from build123d import *

# Parameters (mm, degrees)
F0_R     = 38.1
F1_DEPTH = 76.2
F2_R     = 31.75
F3_DEPTH = 19.05
F4_R     = 5.08
F6_D     = 7.62
F6_DEPTH = 21.59
F6_TIP   = 2.2892789585
F7_D     = 60.96
F7_DEPTH = 55.88
F7_TIP   = 18.314231668


with BuildPart() as f1:
    # F0 (on Front) → F1 (new body)
    with BuildSketch(Plane.XZ):
        Circle(F0_R)
    extrude(amount=F1_DEPTH)

    # F2 (on Front) → F3 (join)
    with BuildSketch(Plane.XZ):
        Circle(F2_R)
    extrude(amount=-F3_DEPTH)

    # F4
    f4_edges = [f1.edges().sort_by_distance(p)[0] for p in [
        (-31.75, 19.05, 0),
        (38.1, -38.1, 0),
        (-38.1, 0, 0),
        (-38.1, -76.2, 0),
    ]]
    fillet(f4_edges, radius=F4_R)

    # F6 (one way)
    with BuildSketch(Plane.XZ):
        with Locations((0, 0)):
            Circle(F6_D / 2)
    extrude(amount=-F6_DEPTH, mode=Mode.SUBTRACT)
    with Locations(Plane.XZ):
        with Locations((0, 0)):
            with Locations((0, 0, -(F6_DEPTH + F6_TIP / 2))):  # 118° drill point
                Cone(0, F6_D / 2, F6_TIP, mode=Mode.SUBTRACT)

    # F7 (one way)
    with BuildSketch(Plane(origin=(0, 0, 0), x_dir=(1, 0, 0), z_dir=(0, 1, 0))):
        with Locations((0, 0)):
            Circle(F7_D / 2)
    extrude(amount=-F7_DEPTH, mode=Mode.SUBTRACT)
    with Locations(Plane(origin=(0, 0, 0), x_dir=(1, 0, 0), z_dir=(0, 1, 0))):
        with Locations((0, 0)):
            with Locations((0, 0, -(F7_DEPTH + F7_TIP / 2))):  # 118° drill point
                Cone(0, F7_D / 2, F7_TIP, mode=Mode.SUBTRACT)


solid = f1.part
Read the model definition and answer for the solid it produces. Units are mm, in the model's axes. A direction names the side the tool comes from. Round coordinates to 2 decimals unless told otherwise and drop trailing zeros. Loops run counter-clockwise (first coordinate to the right, second up) from the corner with the lowest first, then second, coordinate; pieces in that order, holes last.
Q1. Section A-A on y = 6 is taken. Write down the section's boundary in (x, z).
Q2. Consider probe 1 along Z at (x, y) = (0, -40); probe 2 along Z at (x, y) = (0, 14); probe 3 along X at (y, z) = (-23.5, -1). Determine where each line is inside the solid, lowest interval first.
Q3. Determine the mould class of faces 1 (the face through (-30.235, -37.638, -23.183)), 2 (the face through (5.049, -71.014, -1.59)), 3 (the face through (-17, 0, 27)) for opening direction Z: released by +Z, released by -Z, zero draft, split by the parting line, or undercut.
Q4. Each of these flat-tipped pins is pushed along its axis until it touches: pin 1 (4 mm diameter, centred on y = -26, z = -25.5, fed in from -X); pin 2 (10 mm diameter, centred on x = 5, y = -8, fed in from -Z); pin 3 (5 mm diameter, centred on x = -28.5, z = -23.5, fed in from -Y); pin 4 (10 mm diameter, centred on x = 0, z = 0, fed in from +Y). Where does it stop, or does it pass through?
Q5. Which of the six approach directions +Z, -Z, +X, -X, +Y, -Y give full straight-line access (tool end or side, diameter ignored) to faces 4 (the face through (6, 0, 0)), 5 (the face through (-0.83, 9.39, -3.72)), 6 (the face through (0, -76.2, 0))?
Q6. Section B-B on y = -21.5 is taken. Write down the section's boundary in (x, z), and give its area (3 significant figures).
Output:
1. outline: circle Ø63.5 at (0, 0); hole circle Ø7.62 at (0, 0)
2. probe 1: z = -38.1 to -30.48, 30.48 to 38.1
2. probe 2: z = -31.75 to -3.81, 3.81 to 31.75
2. probe 3: x = -38.09 to -30.46, 30.46 to 38.09
3. face 1: split by the parting line
3. face 2: undercut
3. face 3: zero draft
4. pin 1: stops at x = -29.99
4. pin 2: stops at z = -38.1
4. pin 3: stops at y = -76
4. pin 4: stops at y = 19.05
5. face 4: none
5. face 5: +Y
5. face 6: +Z, -Z, +X, -X, -Y
6. outline: circle Ø76.2 at (0, 0); hole circle Ø60.96 at (0, 0)
6. area: 1,640 mm2
